from build123d import *

# Parameters (mm, degrees)
F0_R           = 5.5
F1_DEPTH       = 10
F2_R           = 0.241421
F4_D           = 0.1
F4_CSINK_D     = 10.5
F4_CSINK_ANGLE = 135
F5_DEPTH       = 8


with BuildPart() as f1:
    # F0 (on Top) → F1 (new body)
    with BuildSketch(Plane.XY):
        Circle(F0_R)
    extrude(amount=F1_DEPTH)

    # F2
    f2_edges = [f1.edges().sort_by_distance(p)[0] for p in [
        (-5.5, 0, 10),
    ]]
    fillet(f2_edges, radius=F2_R)

    # F4 (through all)
    with Locations(Plane.XY.offset(10)):
        with Locations((0, 0)):
            CounterSinkHole(F4_D / 2, F4_CSINK_D / 2, counter_sink_angle=F4_CSINK_ANGLE)

    # F0 (on Top) → F5 (join)
    with BuildSketch(Plane.XY):
        Circle(F0_R)
    extrude(amount=F5_DEPTH)


solid = f1.part
Source: CAD feature listing. Evaluate the final solid. Frame: model axes, mm. Round coordinates to 2 decimals unless told otherwise and drop trailing zeros. Order: outer loops, then holes, each group sorted by start corner. A loop starts at its lowest first (then second) coordinate and runs counter-clockwise, first axis right, second up. Notation, with made-up numbers: (36, 32) - (62, 32) arc R23 ccw to (62, 71) - close; hole circle Ø8 at (70, 46.5). An arc over 180 degrees is marked (long way). Use a Markdown table: item, result. Add a question column.
1. First-contact query: pin 1 (5 mm diameter, centred on x = 4.5, z = 3, fed in from +Y); pin 2 (4 mm diameter, centred on x = 3, z = 4, fed in from -Y); pin 3 (0.9 mm diameter, centred on x = 0, y = 0, fed in from +Z); pin 4 (5 mm diameter, centred on y = 0.5, z = 1, fed in from -X). Flat tips, straight axial feed; report the tip coordinate or a pass-through.
2. Line query: probe 1 along X at (y, z) = (3.5, 6.75); probe 2 along Z at (x, y) = (-2.75, 0.75); probe 3 along Z at (x, y) = (-3.5, -1.5). Output: solid intervals per line, ascending.
3. Mould query, pull axis Y, two halves, no side actions, for faces 1 (the cylindrical face through (-1.19, -5.37, 4.81)), 2 (the conical face through (-0.63, 0.2, 8.1)), 3 (the flat face through (0, 0, 0)). Classes: +Y half, -Y half, draft (parallel to the pull), parting line (faces both ways), or undercut.
4. Section query C-C (z = 1.5). Return the cut outline in (x, y), then the cut area to 3 significant figures.
Derived:
| question | item | result |
|---|---|---|
| 1 | pin 1 | y = 5.12 |
| 1 | pin 2 | y = -5.41 |
| 1 | pin 3 | z = 8.01 |
| 1 | pin 4 | x = -5.5 |
| 2 | probe 1 | -4.24 to 4.24 |
| 2 | probe 2 | 0 to 9.01 |
| 2 | probe 3 | 0 to 9.4 |
| 3 | face 1 | parting line |
| 3 | face 2 | undercut |
| 3 | face 3 | draft |
| 4 | outline | circle Ø11 at (0, 0) |
| 4 | area | 95.0 mm2 |
